Could you check a few things on this drawing? It's one solid part, dimensions in mm from its lowest x, y, z. A direction names the side the tool comes from. Give positions to 0.01 mm unless a question says otherwise; leave off trailing zeros. Write each loop counter-clockwise with the first axis right and the second up, starting at its lowest first coordinate (ties: lowest second). Pieces come first, ordered by that corner, then holes.
1. Suppose I cut it at C-C (z = 3.85). Please give me the cut outline in (x, y), and give its area (3 significant figures).
2. Suppose I cut it at B-B (x = 14). Please give me the cut outline in (y, z), and give its area (3 significant figures).
3. On a 3-axis mill with a long thin cutter (end or side, diameter ignored), from which of +Z, -Z, +X, -X, +Y, -Y can I reach the whole of each face in a straight line? I mean the marked faces 4, 5 and 6. Say none if no direction works.
4. If I drill on probe 1 along Z at (x, y) = (1.2, 4.75); probe 2 along Z at (x, y) = (8.25, 4); probe 3 along Y at (x, z) = (3, 4), over which ranges is the centre line in solid material (lowest first)?
5. Thinking about a two-plate mould opening in Y: for the marked faces 1, 2 and 3, which applies, pulls with the +Y half, pulls with the -Y half, needs draft (parallel to the pull), parting line crosses it, or undercut?
6. Suppose I cut it at A-A (y = 4.75). Please give me the cut outline in (x, z).
7. I'm going to push flat-ended pins straight in: pin 1 (1 mm diameter, centred on y = 2.5, z = 4, fed in from -X); pin 2 (1 mm diameter, centred on x = 3.5, z = 2, fed in from -Y); pin 3 (1 mm diameter, centred on x = 8, z = 6, fed in from +Y). Where does each tip first touch, or does it pass through?
8. Suppose I cut it at D-D (x = 3.25). Please give me the cut outline in (y, z).
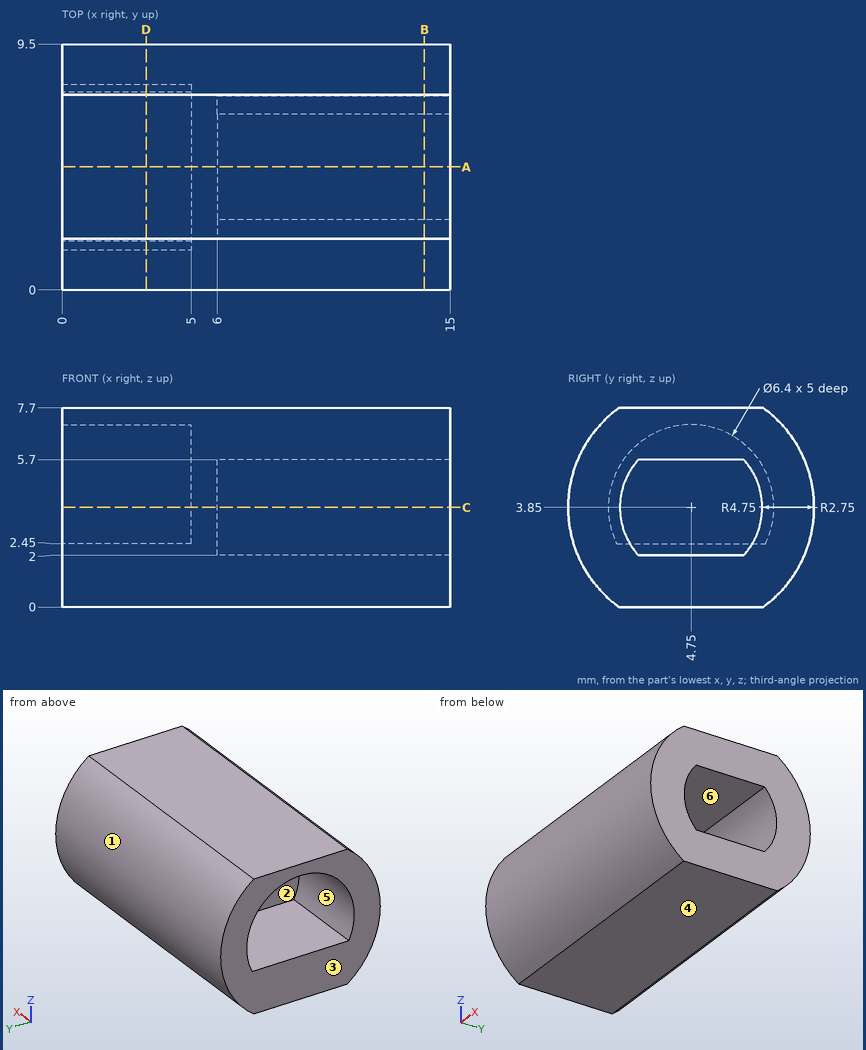
Checks:
1. outline: (0, 0) - (15, 0) - (15, 2) - (6, 2) - (6, 7.5) - (15, 7.5) - (15, 9.5) - (0, 9.5) - (0, 7.95) - (5, 7.95) - (5, 1.55) - (0, 1.55) - close
1. area: 61.0 mm2
2. outline: (1.97, 0) - (7.53, 0) arc R4.75 ccw to (7.53, 7.7) - (1.97, 7.7) arc R4.75 ccw to start; hole (2.72, 2) - (6.78, 2) arc R2.75 ccw to (6.78, 5.7) - (2.72, 5.7) arc R2.75 ccw to start
2. area: 45.4 mm2
3. face 4: -Z, +X, -X, +Y, -Y
3. face 5: -X
3. face 6: +X
4. probe 1: z = 0 to 2.45, 7.05 to 7.7
4. probe 2: z = 0 to 2, 5.7 to 7.7
4. probe 3: y = 0 to 1.55, 7.95 to 9.5
5. face 1: pulls with the +Y half
5. face 2: undercut
5. face 3: needs draft
6. outline: (0, 0) - (15, 0) - (15, 2) - (6, 2) - (6, 5.7) - (15, 5.7) - (15, 7.7) - (0, 7.7) - (0, 7.05) - (5, 7.05) - (5, 2.45) - (0, 2.45) - close
7. pin 1: stops at x = 5
7. pin 2: stops at y = 0.2
7. pin 3: stops at y = 9.2
8. outline: (1.97, 0) - (7.53, 0) arc R4.75 ccw to (7.53, 7.7) - (1.97, 7.7) arc R4.75 ccw to start; hole (1.87, 2.45) - (7.63, 2.45) arc R3.2 ccw (long way) to start
